Part model, mm, in its own coordinate system. A direction names the side the tool comes from. Round coordinates to 2 decimals unless told otherwise and drop trailing zeros. Loops run counter-clockwise (first coordinate to the right, second up) from the corner with the lowest first, then second, coordinate; pieces in that order, holes last. Notation, with made-up numbers: M -30,70.25 L 13,70.25 A22 ccw 13,99.25 Z; hole C -0.5,-23 d7. An arc over 180 degrees is marked long. Put each result on its own line as item: value. Start each with the question number.
1) Probe line 1 along Y through (x, z) = (-2.55, -1.7); line 2 along Y through (x, z) = (-2.55, -0.15); line 3 along Y through (x, z) = (13, 0.75). List the from-to ranges inside material, lowest first.
2) Pull direction X, two halves, no side cores. Call faces 4 (the flat face through (13.15, 5, 3)), 5 (the flat face through (1, 2, -2)), 6 (the cylindrical face through (-3.4, 4.8, -1.2)), 7 (the cylindrical face through (14.87, 4, 7.74)): +X half, -X half, draft (parallel to the pull), parting line (faces both ways), or undercut.
3) Slice it at A-A on x = 14.65. Give the cut face in (y, z) (3 decimals), then the cut area to 3 significant figures.
4) Which spindle directions (+Z, -Z, +X, -X, +Y, -Y) get a long thin tool onto all of the face, cutting with end or side? Do faces 1 (the flat face through (12, 2, 4)), 2 (the flat face through (16, 6, 7)), 3 (the cylindrical face through (-3.049, 3.255, 0.26)). Say none if no direction does.
5) Slice it at B-B on z = 8. Give the cut face in (x, y) (3 decimals).
6) Drop flat-ended pins along their axis: pin 1 Ø7.5 at (x, y) = (-2.55, -5.5) entering from +Z; pin 2 Ø0.8 at (y, z) = (0.5, 0) entering from +X; pin 3 Ø6.5 at (y, z) = (3.5, 6) entering from -X. Give the stop position or say it passes through.
7) Slice it at D-D on z = 2.5. Give the cut face in (x, y).
8) Slice it at C-C on y = -5.5. Give the cut face in (x, z).
```python
from build123d import *

# Parameters (mm, degrees)
SKETCH_1_W                = 14.3
SKETCH_1_H                = 16
EXTRUDE_1_DEPTH           = 1
SKETCH_3_R                = 3
CUT_EXTRUDE_3_DEPTH       = 10
SKETCH_4_R                = 1.25
CUT_EXTRUDE_4_DEPTH       = 2
CHAMFER_2_SIZE            = 3
SKETCH1_W                 = 2
SKETCH1_H                 = 16
EXTRUDE1_DEPTH            = 8
SKETCH2_W                 = 2
SKETCH2_H                 = 16
EXTRUDE2_DEPTH            = 10
SKETCH3_W                 = 14.3
SKETCH3_H                 = 10
EXTRUDE3_DEPTH            = 10
HOLE_WIZARD_M2_5_2_D      = 2.05
HOLE_WIZARD_M2_5_2_DEPTH  = 7.25
HOLE_WIZARD_M2_5_2_TIP    = 0.615882135
CHAMFER1_SIZE             = 3
CHAMFER4_SIZE             = 0.5
EXTRUDE4_DEPTH            = 6
SKETCH7_W                 = 2
SKETCH7_H                 = 6
EXTRUDE5_DEPTH            = 10
CHAMFER5_SIZE             = 0.5
EXTRUDE6_START            = -2
SKETCH8_W                 = 16
SKETCH8_H                 = 16
SKETCH8_R                 = 3
EXTRUDE6_DEPTH            = 2
SKETCH9_R                 = 1.1
EXTRUDE7_DEPTH            = 21.545619971
SKETCH12_W                = 6
SKETCH12_H                = 6
EXTRUDE10_DEPTH           = 0.5
SKETCH13_W                = 8
SKETCH13_H                = 6
EXTRUDE11_DEPTH           = 0.5
SKETCH15_R                = 1.1
SKETCH15_R_2              = 3
EXTRUDE13_DEPTH           = 1
CUT_EXTRUDE_1_DEPTH       = 10
HOLE_WIZARD_1_D           = 2.2
HOLE_WIZARD_1_CBORE_D     = 4.6
HOLE_WIZARD_1_CBORE_DEPTH = 1.5
FILLET_3_R                = 1
SKETCH_12_W               = 8.120884579
SKETCH_12_H               = 6.489865184
CUT_EXTRUDE_2_DEPTH       = 10


with BuildPart() as part:
    # 草图1 → 拉伸1 (new, symmetric)
    with BuildSketch(Plane.XY):
        Rectangle(SKETCH_1_W, SKETCH_1_H)
    extrude(amount=EXTRUDE_1_DEPTH, both=True)

    # 草图3 → 拉伸3 (cut)
    with BuildSketch(Plane(origin=(0, 0, -1), x_dir=(-1, 0, 0), z_dir=(0, 0, -1))):
        with Locations((2.55, 0)):
            Circle(SKETCH_3_R)
    extrude(amount=-CUT_EXTRUDE_3_DEPTH, mode=Mode.SUBTRACT)

    # 草图4 → 拉伸4 (cut)
    with BuildSketch(Plane(origin=(0, 0, -1), x_dir=(-1, 0, 0), z_dir=(0, 0, -1))):
        with Locations((2.55, 5)):
            Circle(SKETCH_4_R)
        with Locations((2.55, -5)):
            Circle(SKETCH_4_R)
    extrude(amount=-CUT_EXTRUDE_4_DEPTH, mode=Mode.SUBTRACT)

    # 倒角2
    chamfer_2_edges = [part.edges().sort_by_distance(p)[0] for p in [
        (-7.15, 8, 0),
        (-7.15, -8, 0),
    ]]
    chamfer(chamfer_2_edges, length=CHAMFER_2_SIZE)

    # Sketch1 → Extrude1 (add)
    with BuildSketch(Plane.XY.offset(1)):
        with Locations((6.15, 0)):
            Rectangle(SKETCH1_W, SKETCH1_H)
    extrude(amount=EXTRUDE1_DEPTH)

    # Sketch2 → Extrude2 (add)
    with BuildSketch(Plane(origin=(7.15, 0, 0), x_dir=(0, 0, -1), z_dir=(1, 0, 0))):
        with Locations((-8, 0)):
            Rectangle(SKETCH2_W, SKETCH2_H)
    extrude(amount=EXTRUDE2_DEPTH)

    # Sketch3 → Extrude3 (cut)
    with BuildSketch(Plane.XZ.offset(8)):
        with Locations((10, 4)):
            Rectangle(SKETCH3_W, SKETCH3_H)
    extrude(amount=-EXTRUDE3_DEPTH, mode=Mode.SUBTRACT)

    # M2.5 螺纹孔2
    with Locations(Plane(origin=(14.65, 5, 9), x_dir=(1, 0, 0), z_dir=(0, 0, 1))):
        with Locations((0, 0)):
            Hole(HOLE_WIZARD_M2_5_2_D / 2, depth=HOLE_WIZARD_M2_5_2_DEPTH)
            with Locations((0, 0, -(HOLE_WIZARD_M2_5_2_DEPTH + HOLE_WIZARD_M2_5_2_TIP / 2))):  # 118° drill point
                Cone(0, HOLE_WIZARD_M2_5_2_D / 2, HOLE_WIZARD_M2_5_2_TIP, mode=Mode.SUBTRACT)

    # Chamfer1
    chamfer1_edges = [part.edges().sort_by_distance(p)[0] for p in [
        (2.85, -8, 0),
    ]]
    chamfer(chamfer1_edges, length=CHAMFER1_SIZE)

    # Chamfer4
    chamfer4_edges = [part.edges().sort_by_distance(p)[0] for p in [
        (15.675, 5, 9),
    ]]
    chamfer(chamfer4_edges, length=CHAMFER4_SIZE)

    # Sketch6 → Extrude4 (add)
    with BuildSketch(Plane(origin=(0, 8, 0), x_dir=(-1, 0, 0), z_dir=(0, 1, 0))):
        Polygon((-10.65, 7), (-12.65, 7), (-12.65, -1), (-7.15, -1), (-5.15, 1), (-10.65, 1), align=None)
    extrude(amount=-EXTRUDE4_DEPTH)

    # Sketch7 → Extrude5 (cut)
    with BuildSketch(Plane.XZ.offset(-2)):
        with Locations((6.15, 4)):
            Rectangle(SKETCH7_W, SKETCH7_H)
    extrude(amount=-EXTRUDE5_DEPTH, mode=Mode.SUBTRACT)

    # Chamfer5
    chamfer5_edges = [part.edges().sort_by_distance(p)[0] for p in [
        (17.15, 8, 8),
        (17.15, 2, 8),
        (5.15, 2, 8),
        (5.15, 8, 8),
    ]]
    chamfer(chamfer5_edges, length=CHAMFER5_SIZE)

    # Sketch8 → Extrude6 (add)
    with BuildSketch(Plane.XY.offset(1).offset(EXTRUDE6_START)):
        with Locations((-2.55, 0)):
            Rectangle(SKETCH8_W, SKETCH8_H)
        with Locations(Location((-2.55, 0, 0), (0, 0, 180))):
            Circle(SKETCH8_R, mode=Mode.SUBTRACT)
    extrude(amount=EXTRUDE6_DEPTH)

    # Sketch9 → Extrude7 (cut, through all)
    with BuildSketch(Plane.XY.offset(1)):
        with Locations((-2.55, -5.5)):
            Circle(SKETCH9_R)
        with Locations((-2.55, 5.5)):
            Circle(SKETCH9_R)
    extrude(amount=-EXTRUDE7_DEPTH, mode=Mode.SUBTRACT)

    # Sketch12 → Extrude10 (add)
    with BuildSketch(Plane.ZY.offset(-10.65)):
        with Locations((4, 5)):
            Rectangle(SKETCH12_W, SKETCH12_H)
    extrude(amount=EXTRUDE10_DEPTH)

    # Sketch13 → Extrude11 (add)
    with BuildSketch(Plane(origin=(12.65, 0, 0), x_dir=(0, 0, -1), z_dir=(1, 0, 0))):
        with Locations((-3, 5)):
            Rectangle(SKETCH13_W, SKETCH13_H)
    extrude(amount=EXTRUDE11_DEPTH)

    # Sketch15 → Extrude13 (add)
    with BuildSketch(Plane(origin=(0, 0, -1), x_dir=(-1, 0, 0), z_dir=(0, 0, -1))):
        Polygon((10.55, -8), (10.55, 8), (-13.15, 8), (-13.15, 2), (-5.45, 2), (-5.45, -8), align=None)
        with Locations(Location((2.55, 5.5, 0), (0, 0, 180))):
            Circle(SKETCH15_R, mode=Mode.SUBTRACT)
        with Locations(Location((2.55, -5.5, 0), (0, 0, 180))):
            Circle(SKETCH15_R, mode=Mode.SUBTRACT)
        with Locations((2.55, 0)):
            Circle(SKETCH15_R_2, mode=Mode.SUBTRACT)
    extrude(amount=EXTRUDE13_DEPTH)

    # 草图9 → 切除-拉伸1 (cut)
    with BuildSketch(Plane(origin=(0, 0, -2), x_dir=(-1, 0, 0), z_dir=(0, 0, -1))):
        with BuildLine():
            Line((-5.45, 0), (-5.45, -9.75102195))
            Line((-5.45, -9.75102195), (10.872695199, -9.75102195))
            Line((10.872695199, -9.75102195), (10.872695199, 8))
            Line((10.872695199, 8), (10.55, 8))
            Line((10.55, 8), (2.55, 8))
            ThreePointArc((2.55, 8), (8.206854249, -5.656854249), (-5.45, 0))
        make_face()
    extrude(amount=-CUT_EXTRUDE_1_DEPTH, mode=Mode.SUBTRACT)

    # 打孔尺寸(%根据)内六角圆柱头螺钉的类型1 (through all)
    with Locations(Plane.XY.offset(1)):
        with Locations((-2.55, 5.5), (-2.55, -5.5)):
            CounterBoreHole(HOLE_WIZARD_1_D / 2, HOLE_WIZARD_1_CBORE_D / 2, HOLE_WIZARD_1_CBORE_DEPTH)

    # 圆角3
    fillet_3_edges = [part.edges().sort_by_distance(p)[0] for p in [
        (5.45, 2, -0.5),
    ]]
    fillet(fillet_3_edges, radius=FILLET_3_R)

    # 草图12 → 切除-拉伸2 (cut)
    with BuildSketch(Plane(origin=(0, 8, 0), x_dir=(1, 0, 0), z_dir=(0, 1, 0))):
        with Locations((6.089557711, -7.244932592)):
            Rectangle(SKETCH_12_W, SKETCH_12_H)
    extrude(amount=-CUT_EXTRUDE_2_DEPTH, mode=Mode.SUBTRACT)


solid = part.part
```
Recorded:
1. line 1: y = -8 to -6.6, -4.4 to -3, 3 to 4.4, 6.6 to 8
1. line 2: y = -8 to -7.8, -3.2 to -3, 3 to 3.2, 7.8 to 8
1. line 3: y = 2 to 8
2. face 4: +X half
2. face 5: draft
2. face 6: undercut
2. face 7: undercut
3. outline: M 2,7 L 3.975,7 L 3.975,8.5 L 3.475,9 L 2,9 Z; M 6.025,7 L 8,7 L 8,9 L 6.525,9 L 6.025,8.5 Z
3. area: 7.65 mm2
4. face 1: +Z, -Z, +X, -Y
4. face 2: -Z, +X, +Y, -Y
4. face 3: +Z
5. outline: M 10.15,2 L 16.65,2 L 17.15,2.5 L 17.15,7.5 L 16.65,8 L 10.15,8 Z; hole C 14.65,5 d2.05
6. pin 1: stops at z = 1
6. pin 2: stops at x = 5.45
6. pin 3: stops at x = 10.15
7. outline: M 10.15,2 L 13.15,2 L 13.15,8 L 10.15,8 Z
8. outline: M -8.36,-2 L -3.65,-2 L -3.65,-0.5 L -4.85,-0.5 L -4.85,1 L -8.36,1 Z; M -1.45,-2 L 3.26,-2 L 3.26,1 L -0.25,1 L -0.25,-0.5 L -1.45,-0.5 Z
